Verification items for the finished model (mm, model axes). Give positions to 0.01 mm unless a question says otherwise; leave off trailing zeros. Order: outer loops, then holes, each group sorted by start corner. A loop starts at its lowest first (then second) coordinate and runs counter-clockwise, first axis right, second up. Notation, with made-up numbers: (59, 73.5) - (112, 73.5) arc R29 cw to (112, 112.5) - close; hole circle Ø10 at (63, 8). An arc over 180 degrees is marked (long way). Answer as a JSON object with one key per item and string values.
```python
from build123d import *

# Parameters (mm, degrees)
ESQUISSE1_R        = 1.6
BOSS_EXTRU_1_DEPTH = 3


with BuildPart() as part:
    # Esquisse1 → Boss.-Extru.1 (new body)
    with BuildSketch(Plane.XY):
        Polygon((-324.146226634, 21.123080509), (-228.411595335, -6.322621021), (-221.686141291, -8.251113935), (-206.165691337, -12.701531345), (-167.175777529, -12.701531345), (-129.424828406, -12.701531345), (-123.517939729, -11.007758272), (-113.904378452, -8.251113935), (-107.178924408, -6.322621021), (-11.444293109, 21.123080509), (-5.984240232, 18.096325283), (16.733855492, -61.131089881), (13.707363231, -66.591026451), (-42.255771499, -82.638197107), (-48.091810819, -98.561018129), (-85.310364869, -115.48724507), (-102.69792658, -133.444615579), (-108.937044092, -133.542771169), (-132.888887149, -110.350948678), (-202.701632594, -110.350948678), (-226.653475651, -133.542771169), (-232.892593163, -133.444615579), (-250.280154874, -115.48724507), (-287.498708924, -98.561018129), (-293.334748244, -82.638197107), (-349.297882974, -66.591026451), (-352.324375235, -61.131089881), (-329.606279511, 18.096325283), align=None)
        with Locations((-12.000450916, 13.68165837)):
            Circle(ESQUISSE1_R, mode=Mode.SUBTRACT)
        with Locations((-118.757933777, -16.924131519)):
            Circle(ESQUISSE1_R, mode=Mode.SUBTRACT)
        with Locations((9.292284284, -60.574933915)):
            Circle(ESQUISSE1_R, mode=Mode.SUBTRACT)
        with Locations((-53.656180266, -93.401689518)):
            Circle(ESQUISSE1_R, mode=Mode.SUBTRACT)
        with Locations((-105.923928137, -126.713325795)):
            Circle(ESQUISSE1_R, mode=Mode.SUBTRACT)
        with Locations((-131.530967037, -101.880200807)):
            Circle(ESQUISSE1_R, mode=Mode.SUBTRACT)
        with Locations(Location((-204.059552706, -101.880200807, 0), (0, 0, 180))):
            Circle(ESQUISSE1_R, mode=Mode.SUBTRACT)
        with Locations(Location((-229.666591606, -126.713325795, 0), (0, 0, 180))):
            Circle(ESQUISSE1_R, mode=Mode.SUBTRACT)
        with Locations(Location((-281.934339477, -93.401689518, 0), (0, 0, 180))):
            Circle(ESQUISSE1_R, mode=Mode.SUBTRACT)
        with Locations(Location((-344.882804027, -60.574933915, 0), (0, 0, 180))):
            Circle(ESQUISSE1_R, mode=Mode.SUBTRACT)
        with Locations(Location((-216.832585966, -16.924131519, 0), (0, 0, 180))):
            Circle(ESQUISSE1_R, mode=Mode.SUBTRACT)
        with Locations(Location((-323.590068827, 13.68165837, 0), (0, 0, 180))):
            Circle(ESQUISSE1_R, mode=Mode.SUBTRACT)
        with Locations(Location((-167.795259872, -27.605548894, 0), (0, 0, 180))):
            Circle(ESQUISSE1_R, mode=Mode.SUBTRACT)
    extrude(amount=BOSS_EXTRU_1_DEPTH)


solid = part.part
```
(1) Gauge pin test, flat ends, axial feed: pin 1 Ø1 at (x, z) = (-119.5, 2.5) entering from +Y; pin 2 Ø1.9 at (x, y) = (-118.76, -16.92) entering from +Z; pin 3 Ø1 at (x, z) = (-68.5, 1) entering from +Y; pin 4 Ø1 at (y, z) = (-108.5, 2.5) entering from +X. Record the tip position at first contact, or that the pin passes through.
Computed values:
{"pin 1": "stops at y = -9.71", "pin 2": "passes through", "pin 3": "stops at y = 4.91", "pin 4": "stops at x = -68.85"}
(2) Material ranges on line 1 along X through (y, z) = (-127, 0.75); line 2 along Y through (x, z) = (-171.5, 2.8); line 3 along Y through (x, z) = (-325, 1.1), recorded low to high. Write a range as [from, to].
Computed values:
{"line 1": "x = [-239.13, -231.24], [-228.09, -219.9], [-115.69, -107.5], [-104.35, -96.46]", "line 2": "y = [-110.35, -12.7]", "line 3": "y = [-73.56, 12.93], [14.44, 20.65]"}
(3) Section check C-C (x = -72). Record the cut outline in (y, z), then the cut area to 3 significant figures.
Computed values:
{"outline": "(-109.43, 0) - (3.76, 0) - (3.76, 3) - (-109.43, 3) - close", "area": "340 mm²"}
(4) Release check for a two-part mould opening along X. For faces 1 (the flat face through (-165, -55, 0)), 2 (the flat face through (-268.63, -107.14, 1.48)), 3 (the flat face through (-120.745, -122.109, 1.479)), 4 (the flat face through (-214.51, -121.785, 1.479)) record: pulls with the +X half, pulls with the -X half, needs draft (parallel to the pull), parting line crosses it, or undercut.
Computed values:
{"face 1": "needs draft", "face 2": "pulls with the -X half", "face 3": "undercut", "face 4": "undercut"}
(5) Section check A-A (y = 8). Record the cut outline in (x, z), then the cut area to 3 significant figures.
Computed values:
{"outline": "(-332.5, 0) - (-278.37, 0) - (-278.37, 3) - (-332.5, 3) - close; (-57.22, 0) - (-3.09, 0) - (-3.09, 3) - (-57.22, 3) - close", "area": "325 mm²"}
(6) Section check D-D (y = -75.5). Record the cut outline in (x, z).
Computed values:
{"outline": "(-318.23, 0) - (-17.36, 0) - (-17.36, 3) - (-318.23, 3) - close"}
(7) Section check B-B (z = 0.9). Count the separate pieces of the cut face and the enclosed holes in it, then the cut area to 3 significant figures.
Computed values:
{"separate pieces": "1", "enclosed holes": "13", "area": "36,500 mm²"}
